Read the model definition and answer for the solid it produces. Units are mm, in the model's axes. A direction names the side the tool comes from. Round coordinates to 2 decimals unless told otherwise and drop trailing zeros. Order: outer loops, then holes, each group sorted by start corner. A loop starts at its lowest first (then second) coordinate and runs counter-clockwise, first axis right, second up. Notation, with made-up numbers: (-32, -32.5) -> (22, -32.5) arc R26 cw to (22, -12.5) -> close; hole circle Ø4 at (30.5, -21). An arc over 180 degrees is marked (long way). Answer as a JSON object with one key per item and string values. Group by question number.
Item 1: Consider probe 1 along X at (y, z) = (6.25, -3.5); probe 2 along Z at (x, y) = (1, 1.5); probe 3 along Y at (x, z) = (20, -7.5). Determine where each line is inside the solid, lowest interval first. Write a range as from..to.
Item 2: Section C-C, the plane z = 13.5 is taken. Write down the section's boundary in (x, y).
Item 3: For faces 1 (the flat face through (31.062, 1.237, 0.147)), 2 (the flat face through (34.33, 2.21, 0.35)), 3 (the flat face through (42.395, 9.32, 0.35)), determine the directions among +Z, -Z, +X, -X, +Y, -Y from which every point of the face is accessible in a straight line to the end or side of a thin tool.
Item 4: Given P1, Ø3, axis at y = 9.5, z = 9.5, coming from the -X side; P2, Ø1.5, axis at y = 5, z = -1.5, coming from the -X side; P3, Ø17, axis at x = 16.5, z = -3.5, coming from the +Y side; P4, Ø12, axis at x = 5.5, z = -18.5, coming from the +Y side, each flat-ended and moving along its own axis, determine where each tip first touches the part or whether it passes through.
Item 5: Section B-B, the plane x = 20.5 is taken. Write down the section's boundary in (y, z).
Item 6: Section A-A, the plane z = 5.5 is taken. Write down the section's boundary in (x, y) (1 decimal).
from build123d import *

# Parameters (mm, degrees)
EXTRUDE_THIN1_DEPTH = 10.5
FILLET1_R           = 2
FILLET2_R           = 2
SKETCH3_W           = 50
SKETCH3_H           = 5
BOSS_EXTRUDE1_DEPTH = 20


with BuildPart() as part:
    # Sketch1 → Extrude-Thin1 (new body, symmetric)
    with BuildSketch(Plane.XY):
        with BuildLine():
            ThreePointArc((-14.244997998, 5), (-5.350470229, 7.548509256), (0, 0))
            Line((0, 0), (28, 0))
            Line((28, 0), (52.755002002, 10))
            Line((52.755002002, 10), (52.193172773, 11.390808368))
            Line((52.193172773, 11.390808368), (27.708474677, 1.5))
            Line((27.708474677, 1.5), (1.38083152, 1.5))
            ThreePointArc((1.38083152, 1.5), (-5.573468314, 9.184875828), (-15.415935123, 5.9375))
            Line((-15.415935123, 5.9375), (-14.244997998, 5))
        make_face()
    extrude(amount=EXTRUDE_THIN1_DEPTH, both=True)

    # Fillet1
    fillet1_edges = [part.edges().sort_by_distance(p)[0] for p in [
        (0, 0, 0),
    ]]
    fillet(fillet1_edges, radius=FILLET1_R)

    # Fillet2
    fillet2_edges = [part.edges().sort_by_distance(p)[0] for p in [
        (1.38083152, 1.5, 0),
    ]]
    fillet(fillet2_edges, radius=FILLET2_R)

    # Sketch3 → Boss-Extrude1 (add)
    with BuildSketch(Plane(origin=(48.826887199, 19.72404898, 0), x_dir=(0, 0, -1), z_dir=(0.927205579, 0.374552819, 0))):
        with Locations((0, -9.737478938)):
            Rectangle(SKETCH3_W, SKETCH3_H)
    extrude(amount=-BOSS_EXTRUDE1_DEPTH)


solid = part.part
Values found:
{
 "1": {"probe 1": "-15.15..-12.99, -3.01..-0.85, 34.79..48.14", "probe 2": "-10.5..10.5", "probe 3": "0..1.5"},
 "2": {"outline": "(32.99, 5.52) -> (34.87, 0.89) -> (53.41, 8.38) -> (51.54, 13.01) -> close"},
 "3": {"face 1": "+Z, -Z, -Y", "face 2": "none", "face 3": "+Z, -Z, +Y"},
 "4": {"P1": "x = -13.12", "P2": "x = -15.18", "P3": "y = 1.5", "P4": "through"},
 "5": {"outline": "(0, -10.5) -> (1.5, -10.5) -> (1.5, 10.5) -> (0, 10.5) -> close"},
 "6": {"outline": "(-15.4, 5.9) -> (-14.2, 5) arc R8 cw to (-0.2, 1.6) arc R2 ccw to (1.8, 0) -> (28, 0) -> (34.2, 2.5) -> (34.9, 0.9) -> (53.4, 8.4) -> (51.5, 13) -> (33, 5.5) -> (33.6, 3.9) -> (27.7, 1.5) -> (3, 1.5) arc R2 cw to (1, 2.9) arc R9.5 ccw to start"}
}
